Could you check a few things on this model? Use its own coordinates, in mm. A direction names the side the tool comes from. Coordinates: 2 decimals unless noted, no trailing zeros. Write each loop counter-clockwise with the first axis right and the second up, starting at its lowest first coordinate (ties: lowest second). Pieces come first, ordered by that corner, then holes.
```python
from build123d import *

# Parameters (mm, degrees)
F1_DEPTH  = 28
F2_W      = 45
F2_H      = 5
F3_DEPTH  = 50
F5_DEPTH  = 28.001
F7_DEPTH  = 28
F8_W      = 37.4603138711
F8_H      = 12
F9_DEPTH  = 32.99
F10_W     = 55
F10_H     = 10.051137104
F11_DEPTH = 25
F12_R     = 2.5
F13_DEPTH = 10.052137104
F14_R     = 1.3
F15_DEPTH = 25


with BuildPart() as f1:
    # F0 (on Top) → F1 (new body)
    with BuildSketch(Plane.XY):
        Polygon((93.79, 0), (0, 0), (0, 10), (-10, 10), (-10, -10), (103.79, -10), (103.79, 126.89), (148.79, 126.89), (148.79, 136.89), (93.79, 136.89), (93.79, 103.9), (-10, 103.9), (-10, 83.9), (0, 83.9), (0, 93.9), (93.79, 93.9), align=None)
    extrude(amount=-F1_DEPTH)

    # F2 (on face) → F3 (join)
    with BuildSketch(Plane.XZ.offset(-126.89)):
        with Locations((126.29, -2.5)):
            Rectangle(F2_W, F2_H)
        with Locations((126.29, -25.5)):
            Rectangle(F2_W, F2_H)
    extrude(amount=F3_DEPTH)

    # F4 (on face) → F5 (cut, through all)
    with BuildSketch(Plane(origin=(0, 0, -28), x_dir=(1, 0, 0), z_dir=(0, 0, -1))):
        Polygon((105.9448644519, -76.89), (103.79, -76.89), (148.79, -126.838862896), (148.79, -76.89), align=None)
    extrude(amount=-F5_DEPTH, mode=Mode.SUBTRACT)

    # F6 (on face) → F7 (join)
    with BuildSketch(Plane.XY):
        Polygon((93.79, 103.9), (93.79, 136.89), (60.8, 103.9), align=None)
    extrude(amount=-F7_DEPTH)

    # F8 (on face) → F9 (cut)
    with BuildSketch(Plane(origin=(0, 136.89, 0), x_dir=(-1, 0, 0), z_dir=(0, 1, 0))):
        with Locations((-75.0598430644, -14)):
            Rectangle(F8_W, F8_H)
    extrude(amount=-F9_DEPTH, mode=Mode.SUBTRACT)

    # F10 (on face) → F11 (join)
    with BuildSketch(Plane(origin=(0, 0, -28), x_dir=(1, 0, 0), z_dir=(0, 0, -1))):
        with Locations((121.29, -131.864431448)):
            Rectangle(F10_W, F10_H)
    extrude(amount=F11_DEPTH)

    # F12 (on face) → F13 (cut, through all)
    with BuildSketch(Plane.XZ.offset(-126.838862896)):
        with Locations((126.29, -14)):
            Circle(F12_R)
        with Locations((126.29, -44)):
            Circle(F12_R)
    extrude(amount=-F13_DEPTH, mode=Mode.SUBTRACT)

    # F14 (on face) → F15 (cut)
    with BuildSketch(Plane(origin=(-10, 0, 0), x_dir=(0, -1, 0), z_dir=(-1, 0, 0))):
        with Locations((-96.9, -7)):
            Circle(F14_R)
        with Locations((-96.9, -21)):
            Circle(F14_R)
        with Locations((3, -7)):
            Circle(F14_R)
        with Locations((3, -21)):
            Circle(F14_R)
    extrude(amount=-F15_DEPTH, mode=Mode.SUBTRACT)


solid = f1.part
```
1. On a 3-axis mill with a long thin cutter (end or side, diameter ignored), from which of +Z, -Z, +X, -X, +Y, -Y can I reach the whole of each face in a straight line? I mean faces 1 (the face through (93.79, 121, -14)), 2 (the face through (125.975, 101.515, -25.535)), 3 (the face through (93.79, 132, -40)), 4 (the face through (103.79, 42, -14)), 5 (the face through (-5, 83.9, -14)). Say none if no direction works.
Verdict:
face 1: -X, +Y
face 2: +Z, -Z, +X, -Y
face 3: -Z, -X, +Y, -Y
face 4: +X, -Y
face 5: +Z, -Z, -X
2. For pin 1 (2 mm diameter, centred on x = 12.5, z = -19, fed in from +Y); pin 2 (11 mm diameter, centred on y = 3.5, z = -18.5, fed in from +X); pin 3 (12 mm diameter, centred on x = 80.5, z = -9, fed in from +Y), each with a flat end and sliding along its axis, tell me the tip position at first contact or that it passes through.
Verdict:
pin 1: stops at y = 103.9
pin 2: stops at x = 103.79
pin 3: stops at y = 129.52
3. I want a section at C-C on x = 126.29. Please give me the cut outline in (y, z), plus the area to 3 significant figures.
Verdict:
outline: (101.86, -28) - (126.84, -28) - (126.84, -41.5) - (136.89, -41.5) - (136.89, -16.5) - (126.89, -16.5) - (126.89, -23) - (101.86, -23) - close; (101.86, -5) - (126.89, -5) - (126.89, -11.5) - (136.89, -11.5) - (136.89, 0) - (101.86, 0) - close; (126.84, -53) - (136.89, -53) - (136.89, -46.5) - (126.84, -46.5) - close
area: 681 mm2
4. If we mould it in two halves opening along Y, with no side actions, what happens to faces 6 (the face through (121, 126.839, -40)), 7 (the face through (93.79, 48, -14)), 8 (the face through (69, 96, 0))? For each: pulls with the +Y half, pulls with the -Y half, needs draft (parallel to the pull), parting line crosses it, or undercut.
Verdict:
face 6: pulls with the -Y half
face 7: undercut
face 8: needs draft
5. Please list where these lines run through material, in increasing order: line 1 along Z through (x, y) = (3.75, 96.9); line 2 along Z through (x, y) = (126.29, 130.25); line 3 along Y through (x, z) = (63, -10).
Verdict:
line 1: z = -28 to -22.3, -19.7 to -8.3, -5.7 to 0
line 2: z = -53 to -46.5, -41.5 to -16.5, -11.5 to 0
line 3: y = -10 to 0, 93.9 to 103.9
6. I want a section at B-B on z = -44. Please give me the cut outline in (x, y), plus the area to 3 significant figures.
Verdict:
outline: (93.79, 126.84) - (123.79, 126.84) - (123.79, 136.89) - (93.79, 136.89) - close; (128.79, 126.84) - (148.79, 126.84) - (148.79, 136.89) - (128.79, 136.89) - close
area: 503 mm2
7. I want a section at D-D on y = 65.5. Please give me the cut outline in (x, z).
Verdict:
outline: (93.79, -28) - (103.79, -28) - (103.79, 0) - (93.79, 0) - close
8. I want a section at A-A on x = 32. Please give me the cut outline in (y, z), plus the area to 3 significant figures.
Verdict:
outline: (-10, -28) - (0, -28) - (0, 0) - (-10, 0) - close; (93.9, -28) - (103.9, -28) - (103.9, 0) - (93.9, 0) - close
area: 560 mm2
